Input: part model. Units: mm. Frame: model coordinates. Face numbers are marked on the shaded views. A direction names the side the tool comes from. Give positions to 0.01 mm unless a question says otherwise; leave off trailing zeros. Write each loop counter-clockwise with the first axis right and the second up, starting at its lowest first coordinate (ties: lowest second). Pieces come first, ordered by that corner, then holes. Notation, with made-up numbers: (7, 46) - (21, 46) arc R24 ccw to (21, 65) - close; hole circle Ø5 at (-6, -14). An arc over 180 degrees is marked (long way). Use a Markdown table: item, result. Add a question column.
1. Pin query (flat end, axial travel): pin 1 (8 mm diameter, centred on x = 46, y = 115.5, fed in from -Z); pin 2 (11 mm diameter, centred on x = 17, y = 116.5, fed in from +Z); pin 3 (1.5 mm diameter, centred on y = 143.5, z = 42.5, fed in from +X). Return the tip coordinate at first contact, or that it passes through.
2. Section query A-A, the plane y = 32. Return loops of the section in (x, z), plus the area to 3 significant figures.
3. Material intervals for probe 1 along X at (y, z) = (83, 6.5); probe 2 along X at (y, z) = (44.5, 70); probe 3 along X at (y, z) = (85, 30), sorted ascending.
4. Section query C-C, the plane x = 72. Return loops of the section in (y, z), plus the area to 3 significant figures.
5. Set-up query: the marked faces 4, 5 and 6. Return all of +Z, -Z, +X, -X, +Y, -Y with unobstructed straight access to the full face (end or side cutting, diameter ignored); none if empty.
6. Mould query, pull axis Y, two halves, no side actions, for the marked faces 1, 2 and 3. Classes: released by +Y, released by -Y, zero draft, split by the parting line, or undercut.
7. Section query B-B, the plane z = 22. Return loops of the section in (x, y).
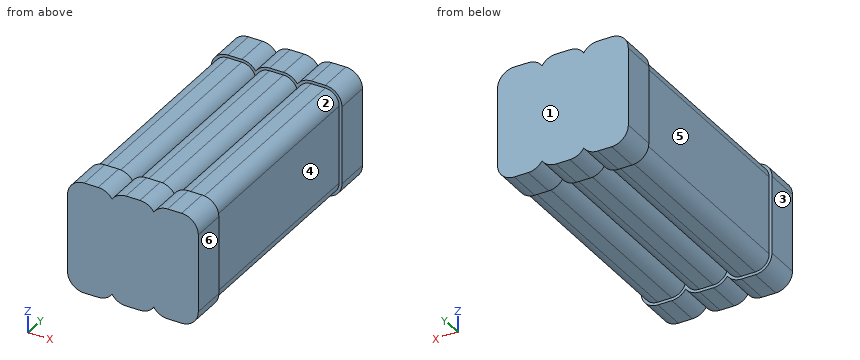
```python
from build123d import *

# Parameters (mm, degrees)
F0_W     = 100
F0_H     = 76
F1_DEPTH = 30
F2_R     = 10
F5_W     = 115
F5_H     = 96
F5_W_2   = 100
F5_H_2   = 56
F6_DEPTH = 30
F8_DEPTH = 25


with BuildPart() as f1:
    # F0 (on Right) → F1 (new body)
    with BuildSketch(Plane.YZ):
        with Locations((50, 38)):
            Rectangle(F0_W, F0_H)
    extrude(amount=F1_DEPTH)

    # F2
    f2_edges = [f1.edges().sort_by_distance(p)[0] for p in [
        (30, 50, 76),
        (0, 50, 76),
        (30, 50, 0),
        (0, 50, 0),
    ]]
    fillet(f2_edges, radius=F2_R)

    # F3: F1 across face


with BuildPart() as f1_1:
    add(f1.part)
    add(f1.part.mirror(Plane(origin=(30, 50, 38), x_dir=(0, 1, 0), z_dir=(1, 0, 0))))

    # F4: F1 across face


with BuildPart() as f1_2:
    add(f1_1.part)
    add(f1_1.part.mirror(Plane(origin=(60, 50, 38), x_dir=(0, 1, 0), z_dir=(1, 0, 0))))

    # F5 (on face) → F6 (cut)
    with BuildSketch(Plane.YZ.offset(120)):
        with Locations((52.5, 38)):
            Rectangle(F5_W, F5_H)
        with Locations((50, 38)):
            Rectangle(F5_W_2, F5_H_2, mode=Mode.SUBTRACT)
        with Locations((50, 38)):
            Rectangle(F5_W_2, F5_H_2)
    extrude(amount=-F6_DEPTH, mode=Mode.SUBTRACT)

    # F7 (on face) → F8 (join)
    with BuildSketch(Plane.XZ):
        with BuildLine():
            ThreePointArc((60, 3.3667504193), (64.3254513381, -0.5735281474), (70, -2))
            Line((70, -2), (80, -2))
            ThreePointArc((80, -2), (88.4852813742, 1.5147186258), (92, 10))
            Line((92, 10), (92, 66))
            ThreePointArc((92, 66), (88.4852813742, 74.4852813742), (80, 78))
            Line((80, 78), (70, 78))
            ThreePointArc((70, 78), (64.3254513381, 76.5735281474), (60, 72.6332495807))
            ThreePointArc((60, 72.6332495807), (55.6745486619, 76.5735281474), (50, 78))
            Line((50, 78), (40, 78))
            ThreePointArc((40, 78), (34.3254513381, 76.5735281474), (30, 72.6332495807))
            ThreePointArc((30, 72.6332495807), (25.6745486619, 76.5735281474), (20, 78))
            Line((20, 78), (10, 78))
            ThreePointArc((10, 78), (1.5147186258, 74.4852813742), (-2, 66))
            Line((-2, 66), (-2, 10))
            ThreePointArc((-2, 10), (1.5147186258, 1.5147186258), (10, -2))
            Line((10, -2), (20, -2))
            ThreePointArc((20, -2), (25.6745486619, -0.5735281474), (30, 3.3667504193))
            ThreePointArc((30, 3.3667504193), (34.3254513381, -0.5735281474), (40, -2))
            Line((40, -2), (50, -2))
            ThreePointArc((50, -2), (55.6745486619, -0.5735281474), (60, 3.3667504193))
        make_face()
        with BuildLine():
            ThreePointArc((0, 66), (2.9289321881, 73.0710678119), (10, 76))
            Line((10, 76), (20, 76))
            ThreePointArc((20, 76), (27.0710678119, 73.0710678119), (30, 66))
            ThreePointArc((30, 66), (32.9289321881, 73.0710678119), (40, 76))
            Line((40, 76), (50, 76))
            ThreePointArc((50, 76), (57.0710678119, 73.0710678119), (60, 66))
            ThreePointArc((60, 66), (62.9289321881, 73.0710678119), (70, 76))
            Line((70, 76), (80, 76))
            ThreePointArc((80, 76), (87.0710678119, 73.0710678119), (90, 66))
            Line((90, 66), (90, 10))
            ThreePointArc((90, 10), (87.0710678119, 2.9289321881), (80, 0))
            Line((80, 0), (70, 0))
            ThreePointArc((70, 0), (62.9289321881, 2.9289321881), (60, 10))
            ThreePointArc((60, 10), (57.0710678119, 2.9289321881), (50, 0))
            Line((50, 0), (40, 0))
            ThreePointArc((40, 0), (32.9289321881, 2.9289321881), (30, 10))
            ThreePointArc((30, 10), (27.0710678119, 2.9289321881), (20, 0))
            Line((20, 0), (10, 0))
            ThreePointArc((10, 0), (2.9289321881, 2.9289321881), (0, 10))
            Line((0, 10), (0, 66))
        make_face(mode=Mode.SUBTRACT)
    extrude(amount=-F8_DEPTH)

    # F9: F1 across face


with BuildPart() as f1_3:
    add(f1_2.part)
    add(f1_2.part.mirror(Plane(origin=(45, 100, 38), x_dir=(-1, 0, 0), z_dir=(0, 1, 0))))


solid = f1_3.part
```
Result sheet:
| question | item | result |
|---|---|---|
| 1 | pin 1 | stops at z = 0 |
| 1 | pin 2 | stops at z = 76 |
| 1 | pin 3 | stops at x = 90 |
| 2 | outline | (0, 10) arc R10 ccw to (10, 0) - (20, 0) arc R10 ccw to (30, 10) arc R10 ccw to (40, 0) - (50, 0) arc R10 ccw to (60, 10) arc R10 ccw to (70, 0) - (80, 0) arc R10 ccw to (90, 10) - (90, 66) arc R10 ccw to (80, 76) - (70, 76) arc R10 ccw to (60, 66) arc R10 ccw to (50, 76) - (40, 76) arc R10 ccw to (30, 66) arc R10 ccw to (20, 76) - (10, 76) arc R10 ccw to (0, 66) - close |
| 2 | area | 6,580 mm² |
| 3 | probe 1 | x = 0.63 to 29.37, 30.63 to 59.37, 60.63 to 89.37 |
| 3 | probe 2 | x = 0.83 to 29.17, 30.83 to 59.17, 60.83 to 89.17 |
| 3 | probe 3 | x = 0 to 90 |
| 4 | outline | (0, -2) - (25, -2) - (25, 0) - (175, 0) - (175, -2) - (200, -2) - (200, 78) - (175, 78) - (175, 76) - (25, 76) - (25, 78) - (0, 78) - close |
| 4 | area | 15,400 mm² |
| 5 | face 4 | +Z, -Z, +X |
| 5 | face 5 | +Z, -Z, -X |
| 5 | face 6 | +Z, -Z, +X, +Y, -Y |
| 6 | face 1 | released by +Y |
| 6 | face 2 | undercut |
| 6 | face 3 | zero draft |
| 7 | outline | (-2, 0) - (92, 0) - (92, 25) - (90, 25) - (90, 175) - (92, 175) - (92, 200) - (-2, 200) - (-2, 175) - (0, 175) - (0, 25) - (-2, 25) - close |
